For this review, take the finished solid that the model builds, in its own axes (mm). A direction names the side the tool comes from. Coordinates: 2 decimals unless noted, no trailing zeros. Order: outer loops, then holes, each group sorted by start corner. A loop starts at its lowest first (then second) coordinate and runs counter-clockwise, first axis right, second up. Notation, with made-up numbers: (40.25, 54) -> (88.25, 54) arc R30 ccw to (88.25, 79) -> close; hole circle Ø9 at (33, 44.25). An arc over 180 degrees is marked (long way). Return JSON: item names as keys, results as strings. Group by question number.
Item 1: Take a section at D-D (x = 42.75). Write out the cut boundary in (y, z).
Item 2: Insertion check: pin 1 (3.5 mm diameter, centred on x = 42.75, y = 5, fed in from +Z); pin 2 (6 mm diameter, centred on x = 41.5, y = 14.5, fed in from +Z); pin 3 (2.5 mm diameter, centred on x = 2.5, z = 2, fed in from +Y); pin 4 (0.6 mm diameter, centred on y = 9.5, z = 4.5, fed in from -X). Each pin has a flat end and moves straight along its axis. Give the tip position at first contact, or say it passes through.
Item 3: Take a section at B-B (x = 22.75). Write out the cut boundary in (y, z), then the cut area to 3 significant figures.
Item 4: Take a section at C-C (z = 2.3). Count the separate pieces of the cut face and the enclosed holes in it, then the cut area to 3 significant figures.
Item 5: Machinability: for faces 4 (the flat face through (23, 27, 4)), 5 (the flat face through (4, 25, 1)), 6 (the flat face through (42, 25, 1)), 7 (the flat face through (4, 13, 3)), 8 (the flat face through (42, 13, 3)), which of the approach directions +Z, -Z, +X, -X, +Y, -Y give a long, thin tool a straight path to every point of the face, cutting with its end or side? Answer none if there is none.
Item 6: Take a section at A-A (y = 20). Write out the cut boundary in (x, z).
Item 7: Draft analysis for pull direction X (two halves, no side actions). For faces 1 (the flat face through (0, 12, 1)), 2 (the flat face through (22, 12, 0)), 3 (the cylindrical face through (17.222, 25.069, 4.507)), state which applies: +X half, -X half, draft (parallel to the pull), parting line (faces both ways), or undercut.
Item 8: For line 1 along Y through (x, z) = (2.75, 2.2); line 2 along Y through (x, z) = (22.75, 3.85); line 3 along Z through (x, y) = (29.5, 20.75), list the stretches that pass through material, from the lowest coordinate up.
```python
from build123d import *
from build123d.topology import SkipClean

# Parameters (mm, degrees)
ESQUISSE1_W             = 45.5
ESQUISSE1_H             = 25
BOSS_EXTRU_1_DEPTH      = 3
ESQUISSE2_R             = 2
ENL_V_MAT_EXTRU_1_DEPTH = 3
ESQUISSE4_W             = 20
ESQUISSE4_H             = 5
BOSS_EXTRU_2_DEPTH      = 3
ESQUISSE3_R             = 6.5
ENL_V_MAT_EXTRU_2_DEPTH = 55.582506355
CHANFREIN1_SIZE         = 5
BOSS_EXTRU_3_START      = 2
ESQUISSE5_R             = 6.5
BOSS_EXTRU_3_DEPTH      = 2
ESQUISSE6_R             = 7.5
ENL_V_MAT_EXTRU_3_DEPTH = 1


with BuildPart() as part:
    # Esquisse1 → Boss.-Extru.1 (new body)
    with BuildSketch(Plane.XY):
        with Locations((22.75, 12.5)):
            Rectangle(ESQUISSE1_W, ESQUISSE1_H)
    extrude(amount=BOSS_EXTRU_1_DEPTH)

    # Esquisse2 → Enlèv. mat.-Extru.1 (cut)
    with BuildSketch(Plane.XY.offset(3)):
        with Locations((2.75, 20)):
            Circle(ESQUISSE2_R)
        with Locations(Location((42.75, 20, 0), (0, 0, 180))):
            Circle(ESQUISSE2_R)
        with Locations((42.75, 5)):
            Circle(ESQUISSE2_R)
        with Locations(Location((2.75, 5, 0), (0, 0, 180))):
            Circle(ESQUISSE2_R)
    extrude(amount=-ENL_V_MAT_EXTRU_1_DEPTH, mode=Mode.SUBTRACT)

    # Esquisse4 → Boss.-Extru.2 (add)
    with BuildSketch(Plane.XY.offset(3)):
        with Locations((22.75, 27.5)):
            Rectangle(ESQUISSE4_W, ESQUISSE4_H)
    extrude(amount=-BOSS_EXTRU_2_DEPTH)

    # Esquisse3 → Enlèv. mat.-Extru.2 (cut, through all)
    with BuildSketch(Plane.XY.offset(3)):
        with Locations((22.75, 20)):
            Circle(ESQUISSE3_R)
    extrude(amount=-ENL_V_MAT_EXTRU_2_DEPTH, mode=Mode.SUBTRACT)

    # Chanfrein1
    chanfrein1_edges = [part.edges().sort_by_distance(p)[0] for p in [
        (32.75, 25, 1.5),
        (12.75, 25, 1.5),
    ]]
    chamfer(chanfrein1_edges, length=CHANFREIN1_SIZE - 0.0001)  # a hair under: the kernel refuses the full size

    # Esquisse5 → Boss.-Extru.3 (add)
    with SkipClean():  # the faces are left unmerged after this step: merging them gives an invalid solid
        with BuildSketch(Plane.XY.offset(3).offset(BOSS_EXTRU_3_START)):
            Polygon((32.75, 30), (12.75, 30), (7.75, 25), (7.75, 0), (37.75, 0), (37.75, 25), align=None)
            with Locations((22.75, 20)):
                Circle(ESQUISSE5_R, mode=Mode.SUBTRACT)
        extrude(amount=-BOSS_EXTRU_3_DEPTH)

    # Esquisse6 → Enlèv. mat.-Extru.3 (cut)
    with SkipClean():  # the faces are left unmerged after this step: merging them gives an invalid solid
        with BuildSketch(Plane.XY.offset(5)):
            with Locations((22.75, 20)):
                Circle(ESQUISSE6_R)
        extrude(amount=-ENL_V_MAT_EXTRU_3_DEPTH, mode=Mode.SUBTRACT)


solid = part.part
```
Findings below:
{
 "1": {"outline": "(0, 0) -> (3, 0) -> (3, 3) -> (0, 3) -> close; (7, 0) -> (18, 0) -> (18, 3) -> (7, 3) -> close; (22, 0) -> (25, 0) -> (25, 3) -> (22, 3) -> close"},
 "2": {"pin 1": "passes through", "pin 2": "stops at z = 3", "pin 3": "stops at y = 25", "pin 4": "stops at x = 7.75"},
 "3": {"outline": "(0, 0) -> (13.5, 0) -> (13.5, 4) -> (12.5, 4) -> (12.5, 5) -> (0, 5) -> close; (26.5, 0) -> (30, 0) -> (30, 5) -> (27.5, 5) -> (27.5, 4) -> (26.5, 4) -> close", "area": "83.0 mm2"},
 "4": {"separate pieces": "1", "enclosed holes": "5", "area": "1,080 mm2"},
 "5": {"face 4": "+Z", "face 5": "+Z, -Z, -X, +Y", "face 6": "+Z, -Z, +X, +Y", "face 7": "+Z, -X, +Y, -Y", "face 8": "+Z, +X, +Y, -Y"},
 "6": {"outline": "(0, 0) -> (0.75, 0) -> (0.75, 3) -> (0, 3) -> close; (4.75, 0) -> (16.25, 0) -> (16.25, 4) -> (15.25, 4) -> (15.25, 5) -> (7.75, 5) -> (7.75, 3) -> (4.75, 3) -> close; (29.25, 0) -> (40.75, 0) -> (40.75, 3) -> (37.75, 3) -> (37.75, 5) -> (30.25, 5) -> (30.25, 4) -> (29.25, 4) -> close; (44.75, 0) -> (45.5, 0) -> (45.5, 3) -> (44.75, 3) -> close"},
 "7": {"face 1": "-X half", "face 2": "draft", "face 3": "undercut"},
 "8": {"line 1": "y = 0 to 3, 7 to 18, 22 to 25", "line 2": "y = 0 to 13.5, 26.5 to 30", "line 3": "z = 0 to 4"}
}
